Geometry check sheet. Reference: the model listing, model coordinates, mm. Coordinates: 2 decimals unless noted, no trailing zeros. Write each loop counter-clockwise with the first axis right and the second up, starting at its lowest first coordinate (ties: lowest second). Pieces come first, ordered by that corner, then holes. Notation, with made-up numbers: (59.25, 64.25) -> (84.25, 64.25) arc R21 cw to (84.25, 87.25) -> close; hole circle Ø10 at (60, -33). An arc over 180 degrees is marked (long way). Put each result on its own line as item: value. Start each with the question number.
from build123d import *

# Parameters (mm, degrees)
MODEL_R             = 7.5
MODEL_R_2           = 3
BOSS_EXTRUDE1_DEPTH = 2


with BuildPart() as part:
    # Model → Boss-Extrude1 (new body)
    with BuildSketch(Plane.XY):
        with BuildLine():
            Line((30.727892071, -23.195832576), (27.969309055, -20.753740651))
            ThreePointArc((27.969309055, -20.753740651), (23.734502764, -21.011453059), (23.992215172, -25.246259349))
            Line((23.992215172, -25.246259349), (26.750798188, -27.688351274))
            ThreePointArc((26.750798188, -27.688351274), (-0.037885337, -38.49998136), (-26.805238954, -27.635650248))
            Line((-26.805238954, -27.635650248), (-24.022447477, -25.18187917))
            ThreePointArc((-24.022447477, -25.18187917), (-23.756401179, -20.947588277), (-27.990692072, -20.68154198))
            Line((-27.990692072, -20.68154198), (-30.773483549, -23.135313057))
            ThreePointArc((-30.773483549, -23.135313057), (-38.5, 0), (-30.773483549, 23.135313057))
            Line((-30.773483549, 23.135313057), (-27.990692072, 20.68154198))
            ThreePointArc((-27.990692072, 20.68154198), (-23.756401179, 20.947588277), (-24.022447477, 25.18187917))
            Line((-24.022447477, 25.18187917), (-26.805238954, 27.635650248))
            ThreePointArc((-26.805238954, 27.635650248), (-0.037885337, 38.49998136), (26.750798188, 27.688351274))
            Line((26.750798188, 27.688351274), (23.992215172, 25.246259349))
            ThreePointArc((23.992215172, 25.246259349), (23.734502764, 21.011453059), (27.969309055, 20.753740651))
            Line((27.969309055, 20.753740651), (30.727892071, 23.195832576))
            ThreePointArc((30.727892071, 23.195832576), (38.5, 0), (30.727892071, -23.195832576))
        make_face()
        Circle(MODEL_R, mode=Mode.SUBTRACT)
        with Locations((0, 25)):
            Circle(MODEL_R_2, mode=Mode.SUBTRACT)
        with Locations((25, 0)):
            Circle(MODEL_R_2, mode=Mode.SUBTRACT)
        with Locations((0, -25)):
            Circle(MODEL_R_2, mode=Mode.SUBTRACT)
        with Locations((-25, 0)):
            Circle(MODEL_R_2, mode=Mode.SUBTRACT)
    extrude(amount=BOSS_EXTRUDE1_DEPTH)


solid = part.part
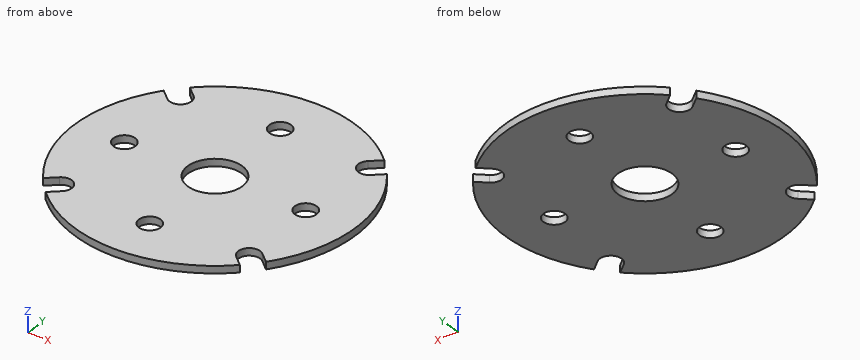
Item 1: Scan lines: line 1 along Y through (x, z) = (0, 1.65); line 2 along X through (y, z) = (2.5, 0.4); line 3 along Y through (x, z) = (-25, 1.15). Record each from-to range of solid material in increasing order. Write a range as [from, to].
Item 2: Section check B-B, the plane z = 1.3. Enter the section's corners in (x, y).
Item 3: Section check D-D, the plane y = 17. Enter the section's corners in (x, z).
Item 4: Go/stop test with flat-tipped pins: P1, Ø5, axis at x = 25, y = 0, coming from the -Z side; P2, Ø1, axis at x = -6, z = 1, coming from the +Y side. Record where each tip stops, or that it passes through.
Item 5: Section check A-A, the plane y = 0. Enter the section's corners in (x, z).
From the geometry:
1. line 1: [-38.5, -28], [-22, -7.5], [7.5, 22], [28, 38.5]
1. line 2: [-38.42, -26.66], [-23.34, -7.07], [7.07, 23.34], [26.66, 38.42]
1. line 3: [-29.28, -26.04], [-20.11, -3], [3, 20.11], [26.04, 29.28]
2. outline: (-30.77, -23.14) -> (-27.99, -20.68) arc R3 cw to (-24.02, -25.18) -> (-26.81, -27.64) arc R38.5 ccw to (26.75, -27.69) -> (23.99, -25.25) arc R3 cw to (27.97, -20.75) -> (30.73, -23.2) arc R38.5 ccw to (30.73, 23.2) -> (27.97, 20.75) arc R3 cw to (23.99, 25.25) -> (26.75, 27.69) arc R38.5 ccw to (-26.81, 27.64) -> (-24.02, 25.18) arc R3 cw to (-27.99, 20.68) -> (-30.77, 23.14) arc R38.5 ccw to start; hole circle Ø6 at (-25, 0); hole circle Ø15 at (0, 0); hole circle Ø6 at (0, -25); hole circle Ø6 at (0, 25); hole circle Ø6 at (25, 0)
3. outline: (-34.54, 0) -> (34.54, 0) -> (34.54, 2) -> (-34.54, 2) -> close
4. P1: through
4. P2: y = 38.11
5. outline: (-38.5, 0) -> (-28, 0) -> (-28, 2) -> (-38.5, 2) -> close; (-22, 0) -> (-7.5, 0) -> (-7.5, 2) -> (-22, 2) -> close; (7.5, 0) -> (22, 0) -> (22, 2) -> (7.5, 2) -> close; (28, 0) -> (38.5, 0) -> (38.5, 2) -> (28, 2) -> close
